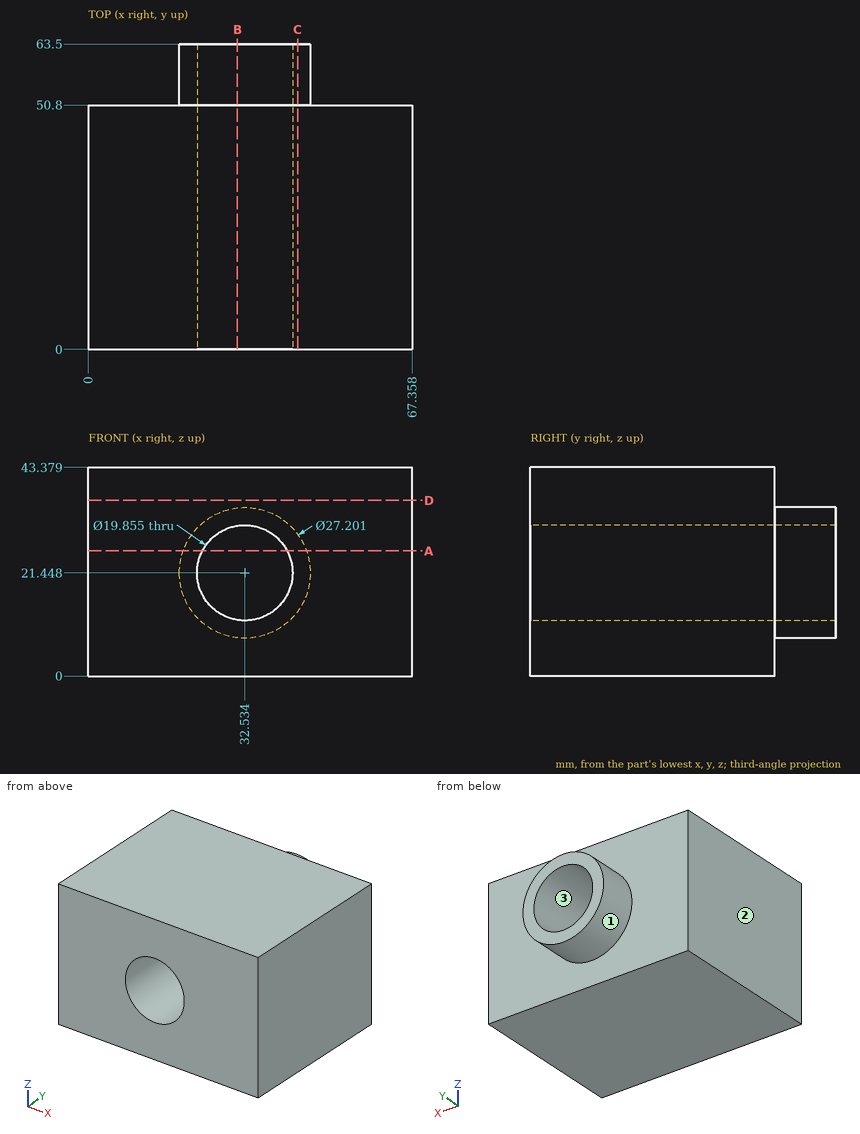
Answer from the drawing. Dimensions are ordinates in mm from the lowest x, y and z of the part. Coordinates: 2 decimals unless noted, no trailing zeros. Order: outer loops, then holes, each group sorted by start corner. A loop starts at its lowest first (then second) coordinate and runs counter-clockwise, first axis right, second up. Notation, with made-up numbers: M -2.75,16 L 53.25,16 A25 ccw 53.25,43 Z; hole C 80.25,15 d11. An arc over 180 degrees is marked long. Put each result on its own line as item: value. Start each with the question number.
Item 1: Section D-D, the plane z = 36.5 is taken. Determine the outline of the cut face in (x, y).
Item 2: Given pin 1 Ø12 at (x, z) = (50.5, 33) entering from +Y, flat-ended and moving along its own axis, determine where the tip first touches the part or whether it passes through.
Item 3: Section B-B, the plane x = 31 is taken. Determine the outline of the cut face in (y, z) (1 decimal), plus the area to 3 significant figures.
Item 4: Consider probe 1 along Y at (x, z) = (26, 38); probe 2 along X at (y, z) = (9.5, 21.5); probe 3 along Z at (x, y) = (41, 47) (1 decimal). Determine where each line is inside the solid, lowest interval first. Write a range as [from, to].
Item 5: Section C-C, the plane x = 43.5 is taken. Determine the outline of the cut face in (y, z).
Item 6: The mould has two halves that part along Z. Classify the marked faces 1, 2 and 3: +Z half, -Z half, draft (parallel to the pull), parting line (faces both ways), or undercut.
Item 7: Section A-A, the plane z = 26 is taken. Determine the outline of the cut face in (x, y), plus the area to 3 significant figures.
Computed:
1. outline: M 0,0 L 67.36,0 L 67.36,50.8 L 0,50.8 Z
2. pin 1: stops at y = 50.8
3. outline: M 0,0 L 50.8,0 L 50.8,7.9 L 63.5,7.9 L 63.5,11.6 L 0,11.6 Z; M 0,31.3 L 63.5,31.3 L 63.5,35 L 50.8,35 L 50.8,43.4 L 0,43.4 Z
3. area: 1,300 mm2
4. probe 1: y = [0, 50.8]
4. probe 2: x = [0, 22.61], [42.46, 67.36]
4. probe 3: z = [0, 16.3], [26.6, 43.4]
5. outline: M 0,0 L 50.8,0 L 50.8,13.4 L 63.5,13.4 L 63.5,29.49 L 50.8,29.49 L 50.8,43.38 L 0,43.38 Z
6. face 1: parting line
6. face 2: draft
6. face 3: undercut
7. outline: M 0,0 L 23.71,0 L 23.71,63.5 L 19.72,63.5 L 19.72,50.8 L 0,50.8 Z; M 41.36,0 L 67.36,0 L 67.36,50.8 L 45.35,50.8 L 45.35,63.5 L 41.36,63.5 Z
7. area: 2,630 mm2
